Build history of the part. All positions in model axes, mm. Face numbers are marked on the shaded views. A direction names the side the tool comes from. Give positions to 0.01 mm unless a question says otherwise; leave off trailing zeros. Write each loop counter-clockwise with the first axis right and the second up, starting at its lowest first coordinate (ties: lowest second). Pieces come first, ordered by that corner, then holes. Notation, with made-up numbers: M 52.25,38 L 67.25,38 A14 ccw 67.25,60 Z; hole C -40,81.25 d1. An arc over 180 degrees is marked long. One line per item, written item: value. Start each with the question number.
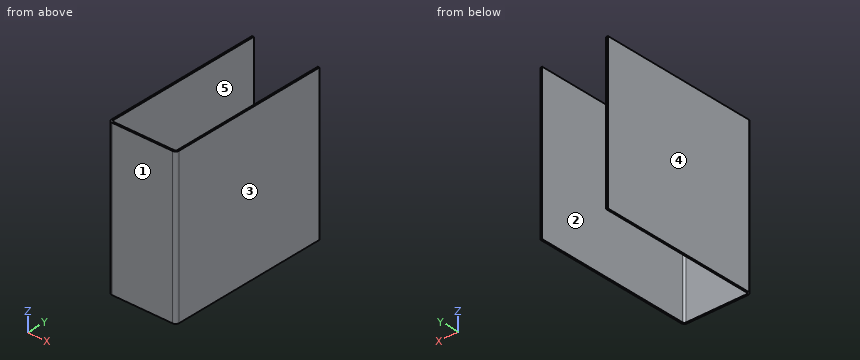
from build123d import *

# Parameters (mm, degrees)
SKETCH_1_W            = 200
SKETCH_1_H            = 480
EXTRUDE_1_DEPTH       = 5
FILLET_1_R            = 5
EXTRUDE_START         = 450
EXTRUDE_3_DEPTH       = 450
CUT_EXTRUDE_START     = -5
CUT_EXTRUDE_2_DEPTH   = 5
SHEET_START           = 5
SHEET_METAL_3_DEPTH   = 450
SHEET_METAL_3_2_DEPTH = 450


# Read off the part's stored shape, not the designer's step: 转换实体3
with BuildPart() as part:
    # 草图1 → 凸台-拉伸1 (new body)
    with BuildSketch(Plane.XY):
        Rectangle(SKETCH_1_W, SKETCH_1_H)
    extrude(amount=EXTRUDE_1_DEPTH)

    # 圆角1
    fillet_1_edges = [part.edges().sort_by_distance(p)[0] for p in [
        (100, -240, 2.5),
        (-100, -240, 2.5),
    ]]
    fillet(fillet_1_edges, radius=FILLET_1_R)

    # 草图4 → 凸台-拉伸3 (add)
    with BuildSketch(Plane.XY.offset(5).offset(EXTRUDE_START)):
        with BuildLine():
            Line((-95, 240), (-95, -235))
            Line((-95, -235), (95, -235))
            Line((95, -235), (95, 240))
            Line((95, 240), (100, 240))
            Line((100, 240), (100, -235))
            ThreePointArc((100, -235), (98.535533906, -238.535533906), (95, -240))
            Line((95, -240), (-95, -240))
            ThreePointArc((-95, -240), (-98.535533906, -238.535533906), (-100, -235))
            Line((-100, -235), (-100, 240))
            Line((-100, 240), (-95, 240))
        make_face()
    extrude(amount=-EXTRUDE_3_DEPTH)

    # Sketch 5 → 切除-拉伸2 (cut)
    with BuildSketch(Plane(origin=(0, 0, 0), x_dir=(-1, 0, 0), z_dir=(0, 0, -1)).offset(CUT_EXTRUDE_START)):
        with BuildLine():
            Line((-95, -240), (95, -240))
            ThreePointArc((95, -240), (98.535533906, -238.535533906), (100, -235))
            Line((100, -235), (100, 240))
            Line((100, 240), (-100, 240))
            Line((-100, 240), (-100, -235))
            ThreePointArc((-100, -235), (-98.535533906, -238.535533906), (-95, -240))
        make_face()
    extrude(amount=CUT_EXTRUDE_2_DEPTH, mode=Mode.SUBTRACT)

    # Sheet Metal 3 outline → Sheet Metal 3 (cut)
    with BuildSketch(Plane.XY.offset(SHEET_START)):
        with BuildLine():
            Line((-95, -240), (-90, -240))
            ThreePointArc((-90, -240), (-97.071067812, -237.071067812), (-100, -230))
            Line((-100, -230), (-100, -235))
            ThreePointArc((-100, -235), (-98.535533906, -238.535533906), (-95, -240))
        make_face()
        with BuildLine():
            ThreePointArc((100, -230), (97.071067812, -237.071067812), (90, -240))
            Line((90, -240), (95, -240))
            ThreePointArc((95, -240), (98.535533906, -238.535533906), (100, -235))
            Line((100, -235), (100, -230))
        make_face()
    extrude(amount=SHEET_METAL_3_DEPTH, mode=Mode.SUBTRACT)

    # Sheet Metal 3 2 outline → Sheet Metal 3 2 (add)
    with BuildSketch(Plane.XY.offset(SHEET_START)):
        with BuildLine():
            Line((-95, -235), (-90, -235))
            ThreePointArc((-90, -235), (-93.535533906, -233.535533906), (-95, -230))
            Line((-95, -230), (-95, -235))
        make_face()
        with BuildLine():
            ThreePointArc((95, -230), (93.535533906, -233.535533906), (90, -235))
            Line((90, -235), (95, -235))
            Line((95, -235), (95, -230))
        make_face()
    extrude(amount=SHEET_METAL_3_2_DEPTH)


solid = part.part
1) Mould opens along X. For the marked faces 3, 4 and 5 say: released by +X, released by -X, zero draft, split by the parting line, or undercut.
2) Band-saw the part on B-B (z = 255). List the corners of the cut face in (x, y).
3) Probe line 1 along X through (y, z) = (-44, 306); line 2 along Y through (x, z) = (49.5, 299). List the from-to ranges inside material, lowest first. Write a range as from..to.
4) Drop a flat-ended pin along its axis: P1, Ø3, axis at x = 69.5, z = 168, coming from the +Y side. Give the stop position or say it passes through.
5) Tool access for the marked faces 1 and 2: list every direction of +Z, -Z, +X, -X, +Y, -Y with a clear straight run to the whole face (end or side of a thin tool).
6) Band-saw the part on A-A (y = 127). List the corners of the cut face in (x, z).
7) Band-saw the part on C-C (x = 80.5). List the corners of the cut face in (y, z).
Model answer:
1. face 3: released by +X
1. face 4: released by -X
1. face 5: undercut
2. outline: M -100,-230 A10 ccw -90,-240 L 90,-240 A10 ccw 100,-230 L 100,240 L 95,240 L 95,-230 A5 cw 90,-235 L -90,-235 A5 cw -95,-230 L -95,240 L -100,240 Z
3. line 1: x = -100..-95, 95..100
3. line 2: y = -240..-235
4. P1: stops at y = -235
5. face 1: +Z, -Z, +X, -X, -Y
5. face 2: +Z, -Z, +Y
6. outline: M -100,5 L -95,5 L -95,455 L -100,455 Z; M 95,5 L 100,5 L 100,455 L 95,455 Z
7. outline: M -240,5 L -235,5 L -235,455 L -240,455 Z
